from build123d import *

# Parameters (mm, degrees)
SKETCH1_R          = 3.175
EXTRUDE1_DEPTH     = 38.1
SKETCH2_W          = 2.380423229
SKETCH2_H          = 32.427702335
EXTRUDE2_DEPTH     = 38.1
SKETCH3_R          = 3.5687
CUT_EXTRUDE1_DEPTH = 2.380423


with BuildPart() as part:
    # Sketch1 → Extrude1 (new body)
    with BuildSketch(Plane.XY):
        with BuildLine():
            Line((214.284444429, 56.4017138), (214.284444429, 94.5017138))
            ThreePointArc((214.284444429, 94.5017138), (203.802872025, 97.073311219), (211.9040212, 89.942543))
            Line((211.9040212, 89.942543), (211.9040212, 56.4017138))
            Line((211.9040212, 56.4017138), (214.284444429, 56.4017138))
        make_face()
        with Locations((208.728194429, 94.5017138)):
            Circle(SKETCH1_R, mode=Mode.SUBTRACT)
    extrude(amount=EXTRUDE1_DEPTH)

    # Sketch2 → Extrude2 (add)
    with BuildSketch(Plane(origin=(0, 0, 0), x_dir=(-1, 0, 0), z_dir=(0, 0, -1))):
        with Locations((-213.094232815, 72.615564968)):
            Rectangle(SKETCH2_W, SKETCH2_H)
    extrude(amount=EXTRUDE2_DEPTH)

    # Sketch3 → Cut-Extrude1 (cut)
    with BuildSketch(Plane.ZY.offset(-211.9040212)):
        with Locations((-25.4, 71.0829138)):
            Circle(SKETCH3_R)
        with Locations((25.4, 71.0829138)):
            Circle(SKETCH3_R)
    extrude(amount=-CUT_EXTRUDE1_DEPTH, mode=Mode.SUBTRACT)


solid = part.part
Input: part model. Units: mm. Frame: model coordinates. A direction names the side the tool comes from. Round coordinates to 2 decimals unless told otherwise and drop trailing zeros. Order: outer loops, then holes, each group sorted by start corner. A loop starts at its lowest first (then second) coordinate and runs counter-clockwise, first axis right, second up. Notation, with made-up numbers: (-1.5, -37.5) - (21.5, -37.5) arc R18 ccw to (21.5, -28.5) - close; hole circle Ø8 at (-26.75, -25.75). An arc over 180 degrees is marked (long way). Use a Markdown table: item, result.
1. First-contact query: pin 1 (1.2 mm diameter, centred on x = 213, z = -12.5, fed in from +Y); pin 2 (17 mm diameter, centred on y = 74.5, z = 7.5, fed in from -X); pin 3 (3.5 mm diameter, centred on x = 211, y = 95, fed in from -Z); pin 4 (4 mm diameter, centred on x = 206.5, z = -3.5, fed in from +Y). Flat tips, straight axial feed; report the tip coordinate or a pass-through.
Evaluation:
| item | result |
|---|---|
| pin 1 | y = 88.83 |
| pin 2 | x = 211.9 |
| pin 3 | z = 0 |
| pin 4 | through |
2. Material intervals for probe 1 along Y at (x, z) = (208.5, 7); probe 2 along X at (y, z) = (68.5, 9); probe 3 along Y at (x, z) = (212.5, 25.4), sorted ascending.
Evaluation:
| item | result |
|---|---|
| probe 1 | 88.95 to 91.33, 97.67 to 100.05 |
| probe 2 | 211.9 to 214.28 |
| probe 3 | 56.4 to 67.51, 74.65 to 98.58 |
3. Section B-B on z = 25.4. State how many separate pieces and enclosed holes the cut face has, then the cut area to 3 significant figures.
Evaluation:
| item | result |
|---|---|
| separate pieces | 2 |
| enclosed holes | 1 |
| area | 131 mm^2 |
4. Section D-D on x = 213.25. Return the cut outline in (y, z).
Evaluation:
| item | result |
|---|---|
| outline | (56.4, -38.1) - (88.83, -38.1) - (88.83, 0) - (97.73, 0) - (97.73, 38.1) - (56.4, 38.1) - close; hole circle Ø7.14 at (71.08, -25.4); hole circle Ø7.14 at (71.08, 25.4) |
5. Section A-A on z = -25.4. Return the cut outline in (x, y).
Evaluation:
| item | result |
|---|---|
| outline | (211.9, 56.4) - (214.28, 56.4) - (214.28, 67.51) - (211.9, 67.51) - close; (211.9, 74.65) - (214.28, 74.65) - (214.28, 88.83) - (211.9, 88.83) - close |
6. Mould query, pull axis Y, two halves, no side actions, for faces 3 (the face through (213, 73, -38.1)), 4 (the face through (211.661, 93.286, 18.783)), 5 (the face through (213, 88.829, -19)). Classes: +Y half, -Y half, draft (parallel to the pull), parting line (faces both ways), or undercut.
Evaluation:
| item | result |
|---|---|
| face 3 | draft |
| face 4 | undercut |
| face 5 | +Y half |
7. Access query for faces 1 (the face through (214.284, 75, 1)), 2 (the face through (211, 92, 0)). Directions: +Z, -Z, +X, -X, +Y, -Y. A direction counts if a zero-diameter tool reaches every point of the face in a straight line with its end or side. Return the directions, or none.
Evaluation:
| item | result |
|---|---|
| face 1 | +Z, -Z, +X, +Y, -Y |
| face 2 | -Z, +X, -X, +Y |
8. Section C-C on x = 207. Return the cut outline in (y, z), then the cut area to 3 significant figures.
Evaluation:
| item | result |
|---|---|
| outline | (89.22, 0) - (91.84, 0) - (91.84, 38.1) - (89.22, 38.1) - close; (97.17, 0) - (99.78, 0) - (99.78, 38.1) - (97.17, 38.1) - close |
| area | 199 mm^2 |
